Read the model definition and answer for the solid it produces. Units are mm, in the model's axes. Coordinates: 2 decimals unless noted, no trailing zeros. Write each loop counter-clockwise with the first axis right and the second up, starting at its lowest first coordinate (ties: lowest second). Pieces come first, ordered by that corner, then holes. Notation, with made-up numbers: M -13,42 L 1,42 A21 cw 1,77 Z; hole C -3,39 d1. An arc over 180 degrees is marked long. Write item = value, one per line.
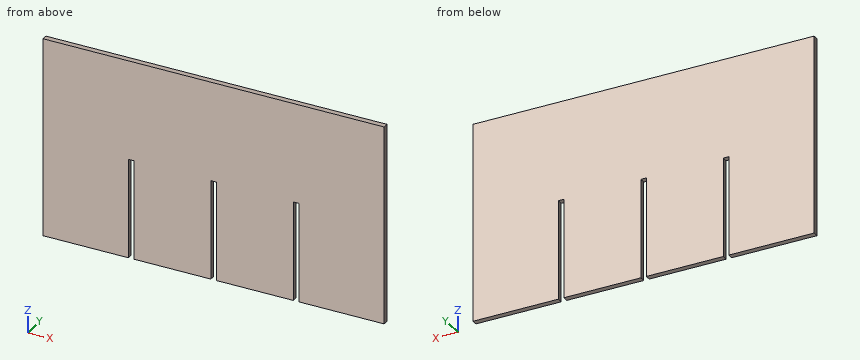
Autodesk Inventor part; units mm, degrees
ref_plane "YZ Plane" through (0, 0, 0) normal (1, 0, 0) x (0, 1, 0)
ref_plane "XZ Plane" through (0, 0, 0) normal (0, 1, 0) x (-1, 0, 0)
ref_plane "XY Plane" through (0, 0, 0) normal (0, 0, 1) x (1, 0, 0)
sketch "Sketch1" plane through (0, 0, 0) normal (0, 1, 0) x (-1, 0, 0)
  line L0 (163.957, -96.9264) -> (-229.743, -96.9264)
  line L1 (-229.743, -96.9264) -> (-229.743, 131.6736)
  line L2 (-229.743, 131.6736) -> (163.957, 131.6736)
  line L3 (163.957, 131.6736) -> (163.957, -96.9264)
  point P0 (0, 0)
  dimension "d0" = 228.6
  dimension "d1" = 393.7
extrude "Board" add sketch "Sketch1" along normal blind 6.35
sketch "Sketch2" plane through (0, 6.35, 0) normal (0, 1, 0) x (1, 0, 0)
  line L0 (-65.532, 96.9264) -> (-59.182, 96.9264)
  line L1 (-59.182, 96.9264) -> (-59.182, -17.3736)
  line L2 (-59.182, -17.3736) -> (-65.532, -17.3736)
  line L3 (-65.532, -17.3736) -> (-65.532, 96.9264)
  line L4 (229.743, 96.9264) -> (-163.957, 96.9264)
  line L5 (-163.957, 96.9264) -> (-163.957, -131.6736)
  line L6 (29.718, 96.9264) -> (36.068, 96.9264)
  line L7 (36.068, 96.9264) -> (36.068, -17.3736)
  line L8 (36.068, -17.3736) -> (29.718, -17.3736)
  line L9 (29.718, -17.3736) -> (29.718, 96.9264)
  line L10 (124.968, 96.9264) -> (131.318, 96.9264)
  line L11 (131.318, 96.9264) -> (131.318, -17.3736)
  line L12 (131.318, -17.3736) -> (124.968, -17.3736)
  line L13 (124.968, -17.3736) -> (124.968, 96.9264)
  line L14 (229.743, -131.6736) -> (229.743, 96.9264)
  point P0 (0, 0)
  dimension "d4" = 6.35
  dimension "d5" = 114.3
  dimension "d6" = 98.425
  dimension "d7" = 6.35
  dimension "d8" = 114.3
  dimension "d10" = 6.35
  dimension "d11" = 114.3
  dimension "d13" = 88.9
  dimension "d14" = 88.9
  dimension "d25" = 98.425
extrude "Stop Dados" cut sketch "Sketch2" against normal blind 6.35
equation "\"d5\" = 0.5 * d0"
equation "\"d8\" = 0.5 * d9"
equation "\"d11\" = 0.5 * d12"
properties part number "Wine Rack Horizontal"
Item 1: A flat-ended cylindrical pin translates along its axis: pin 1 (1.9 mm diameter, centred on x = 33, y = 3, fed in from -Z). Find the tip coordinate at first contact, or state that the pin passes through.
Worked answers:
pin_1 = 17.37
Item 2: Find section A-A (z = 0.5). Determine the outline of the cut face in (x, y), and give its area (3 significant figures).
Worked answers:
outline = M -163.96,0 L -65.53,0 L -65.53,6.35 L -163.96,6.35 Z; M -59.18,0 L 29.72,0 L 29.72,6.35 L -59.18,6.35 Z; M 36.07,0 L 124.97,0 L 124.97,6.35 L 36.07,6.35 Z; M 131.32,0 L 229.74,0 L 229.74,6.35 L 131.32,6.35 Z
area = 2,380 mm²
Item 3: Consider line 1 along X through (y, z) = (4.75, -50); line 2 along Z through (x, y) = (31.5, 2.25). Determine where each line is inside the solid, lowest interval first. Write a range as from..to.
Worked answers:
line_1 = -163.96..-65.53, -59.18..29.72, 36.07..124.97, 131.32..229.74
line_2 = 17.37..131.67
Item 4: Find section B-B (y = 2.75). Determine the outline of the cut face in (x, z).
Worked answers:
outline = M -163.96,-96.93 L -65.53,-96.93 L -65.53,17.37 L -59.18,17.37 L -59.18,-96.93 L 29.72,-96.93 L 29.72,17.37 L 36.07,17.37 L 36.07,-96.93 L 124.97,-96.93 L 124.97,17.37 L 131.32,17.37 L 131.32,-96.93 L 229.74,-96.93 L 229.74,131.67 L -163.96,131.67 Z
